Geometry: see drawing. Coordinates: mm, zero at the bounding-box minimum. A direction names the side the tool comes from. Give positions to 0.01 mm unless a question says otherwise; leave off trailing zeros. Write each loop counter-clockwise with the first axis right and the second up, starting at its lowest first coordinate (ties: lowest second). Pieces come first, ordered by that corner, then holes. Notation, with made-up numbers: (70, 26.5) - (77, 26.5) arc R13 ccw to (77, 35.5) - close; hole circle Ø2 at (66.5, -7.5). An arc over 180 degrees is marked (long way). Return JSON: item names as keys, results as strings.
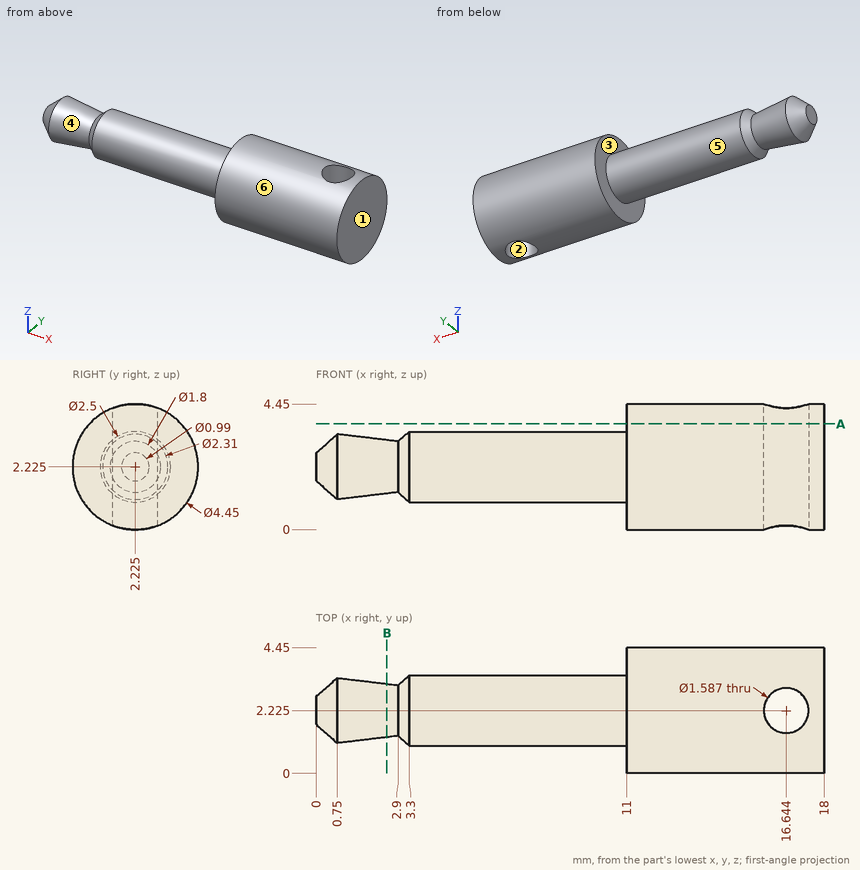
Q1. Mould query, pull axis X, two halves, no side actions, for the marked faces 1, 2 and 3. Classes: pulls with the +X half, pulls with the -X half, needs draft (parallel to the pull), parting line crosses it, or undercut.
Answer key:
{"face 1": "pulls with the +X half", "face 2": "undercut", "face 3": "pulls with the -X half"}
Q2. Set-up query: the marked faces 4, 5 and 6. Return all of +Z, -Z, +X, -X, +Y, -Y with unobstructed straight access to the full face (end or side cutting, diameter ignored); none if empty.
Answer key:
{"face 4": "none", "face 5": "-X", "face 6": "+X, -X"}
Q3. Pin query (flat end, axial travel): P1, Ø1, axis at x = 6, z = 3.5, coming from the +Y side (1 decimal). Return the tip coordinate at first contact, or that it passes through.
Answer key:
{"P1": "stops at y = 3.2"}
Q4. Section query A-A, the plane z = 3.75. Return the cut outline in (x, y) (1 decimal).
Answer key:
{"outline": "(11, 0.6) - (18, 0.6) - (18, 3.8) - (11, 3.8) - close; hole circle Ø1.6 at (16.6, 2.2)"}
Q5. Section query B-B, the plane x = 2.5. Return the cut outline in (y, z) (1 decimal).
Answer key:
{"outline": "circle Ø1.9 at (2.2, 2.2)"}
Q6. Material intervals for probe 1 along X at (y, z) = (2.2, 3.95); probe 2 along X at (y, z) = (0.65, 1.65); probe 3 along Y at (x, z) = (8.5, 2.2) (1 decimal), sorted ascending. Write a range as [from, to].
Answer key:
{"probe 1": "x = [11, 15.85], [17.44, 18]", "probe 2": "x = [11, 18]", "probe 3": "y = [1, 3.5]"}
